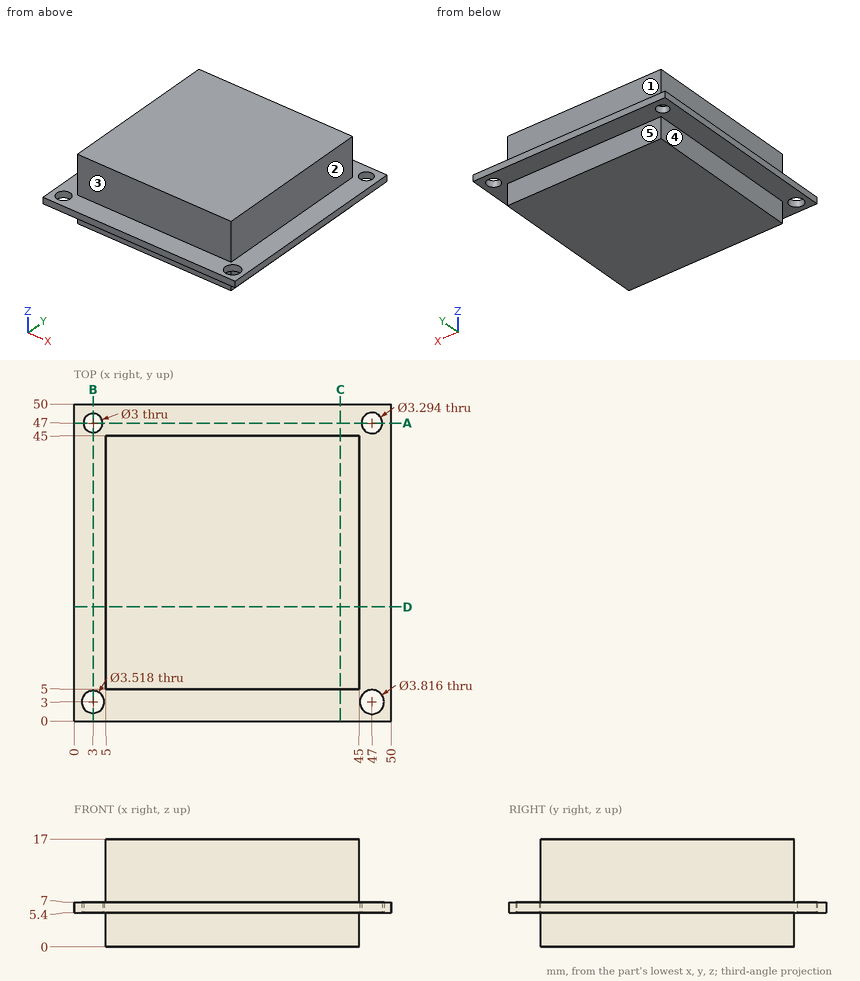
Geometry check sheet. Reference: drawing and pictorial views, mm from the part's lowest x, y, z. A direction names the side the tool comes from. Coordinates: 2 decimals unless noted, no trailing zeros. Order: outer loops, then holes, each group sorted by start corner. A loop starts at its lowest first (then second) coordinate and runs counter-clockwise, first axis right, second up.
Item 1: Section check A-A, the plane y = 47. Enter the section's corners in (x, z).
Filled in:
outline: (0, 5.4) - (1.5, 5.4) - (1.5, 7) - (0, 7) - close; (4.5, 5.4) - (45.35, 5.4) - (45.35, 7) - (4.5, 7) - close; (48.65, 5.4) - (50, 5.4) - (50, 7) - (48.65, 7) - close
Item 2: Section check C-C, the plane x = 42. Enter the section's corners in (y, z).
Filled in:
outline: (0, 5.4) - (5, 5.4) - (5, 0) - (45, 0) - (45, 5.4) - (50, 5.4) - (50, 7) - (45, 7) - (45, 17) - (5, 17) - (5, 7) - (0, 7) - close
Item 3: Material ranges on L1, parallel to Y at x = 3, z = 6.1; L2, parallel to Y at x = 47, z = 6.3; L3, parallel to Y at x = 32, z = 13.25, recorded low to high.
Filled in:
L1: y = 0 to 1.24, 4.76 to 45.5, 48.5 to 50
L2: y = 0 to 1.09, 4.91 to 45.35, 48.65 to 50
L3: y = 5 to 45
Item 4: Depth check by flat-ended pin: pin 1 (6 mm diameter, centred on x = 31, z = 2, fed in from -Y); pin 2 (2 mm diameter, centred on x = 24.5, y = 18.5, fed in from -Z); pin 3 (2 mm diameter, centred on y = 16, z = 15.5, fed in from +X); pin 4 (8 mm diameter, centred on x = 26, z = 11.5, fed in from +Y). Enter the tip coordinate at first touch or a pass-through.
Filled in:
pin 1: stops at y = 5
pin 2: stops at z = 0
pin 3: stops at x = 45
pin 4: stops at y = 45
Item 5: Access from +Z, -Z, +X, -X, +Y, -Y to the whole of each face (thin tool, end or side, straight path). Record for the marked faces 1, 2, 3, 4 and 5.
Filled in:
face 1: +Z, +X, -X, +Y
face 2: +Z, +X, +Y, -Y
face 3: +Z, +X, -X, -Y
face 4: -Z, -X, +Y, -Y
face 5: -Z, +X, -X, +Y
Item 6: Section check B-B, the plane x = 3. Enter the section's corners in (y, z).
Filled in:
outline: (0, 5.4) - (1.24, 5.4) - (1.24, 7) - (0, 7) - close; (4.76, 5.4) - (45.5, 5.4) - (45.5, 7) - (4.76, 7) - close; (48.5, 5.4) - (50, 5.4) - (50, 7) - (48.5, 7) - close
